from build123d import *

# Parameters (mm, degrees)
SKETCH_1_W                   = 160
SKETCH_1_H                   = 120
EXTRUDE_1_DEPTH              = 4
SKETCH_2_R                   = 4
SKETCH_2_R_2                 = 2.65
SKETCH_2_R_3                 = 6.75
CUT_EXTRUDE_1_DEPTH          = 24
CUT_EXTRUDE_2_DEPTH          = 54
SKETCH_5_R                   = 1.525
CUT_EXTRUDE_3_DEPTH          = 54
CUT_EXTRUDE_4_DEPTH          = 84
FILLET_1_R                   = 10
HOLE_WIZARD_M3_1_D           = 3.05
HOLE_WIZARD_M3_1_DEPTH       = 7.5
HOLE_WIZARD_M3_1_CSINK_D     = 6.6
HOLE_WIZARD_M3_1_CSINK_ANGLE = 90
HOLE_WIZARD_M3_1_TIP         = 0.916312444
FILLET_2_R                   = 2


with BuildPart() as part:
    # 草图1 → 凸台-拉伸1 (new body)
    with BuildSketch(Plane.XY):
        Rectangle(SKETCH_1_W, SKETCH_1_H)
    extrude(amount=EXTRUDE_1_DEPTH)

    # 草图2 → 切除-拉伸1 (cut)
    with BuildSketch(Plane(origin=(0, 0, 0), x_dir=(-1, 0, 0), z_dir=(0, 0, -1))):
        with Locations((-47.5, 38)):
            Circle(SKETCH_2_R)
        with Locations((-56.749921469, 44.53912734)):
            Circle(SKETCH_2_R_2)
        with Locations((-69.194904497, 52.913039057)):
            Circle(SKETCH_2_R_2)
        with Locations((-27.711627738, 25)):
            Circle(SKETCH_2_R_2)
        with Locations((-10, 25)):
            Circle(SKETCH_2_R_3)
    cut_extrude_1 = extrude(amount=-CUT_EXTRUDE_1_DEPTH, mode=Mode.SUBTRACT)

    # 镜向1: 切除-拉伸1 across plane
    add(cut_extrude_1.mirror(Plane(origin=(0, 0, 0), x_dir=(0, 0, 1), z_dir=(1, 0, 0))), mode=Mode.SUBTRACT)

    # 草图3 → 切除-拉伸2 (cut)
    with BuildSketch(Plane(origin=(0, 0, 0), x_dir=(-1, 0, 0), z_dir=(0, 0, -1))):
        Polygon((-61.851610318, 60), (-40.030198451, 45), (40.030198451, 45), (61.851610318, 60), align=None)
    extrude(amount=-CUT_EXTRUDE_2_DEPTH, mode=Mode.SUBTRACT)

    # 草图5 → 切除-拉伸3 (cut)
    with BuildSketch(Plane(origin=(0, 0, 0), x_dir=(-1, 0, 0), z_dir=(0, 0, -1))):
        with Locations((-20.859650045, 35.859650045)):
            Circle(SKETCH_5_R)
        with Locations((-20.859650045, -5.859650045)):
            Circle(SKETCH_5_R)
        with Locations((20.859650045, -5.859650045)):
            Circle(SKETCH_5_R)
        with Locations((20.859650045, 35.859650045)):
            Circle(SKETCH_5_R)
    extrude(amount=-CUT_EXTRUDE_3_DEPTH, mode=Mode.SUBTRACT)

    # 草图6 → 切除-拉伸4 (cut)
    with BuildSketch(Plane(origin=(0, 0, 0), x_dir=(-1, 0, 0), z_dir=(0, 0, -1))):
        with BuildLine():
            Line((-80, 50), (-28.863438287, -9.71643037))
            ThreePointArc((-28.863438287, -9.71643037), (0, -23), (28.863438287, -9.71643037))
            Line((28.863438287, -9.71643037), (80, 50))
            Line((80, 50), (80, -60))
            Line((80, -60), (-80, -60))
            Line((-80, -60), (-80, 50))
        make_face()
    extrude(amount=-CUT_EXTRUDE_4_DEPTH, mode=Mode.SUBTRACT)

    # 圆角1
    fillet_1_edges = [part.edges().sort_by_distance(p)[0] for p in [
        (-80, 60, 2),
        (80, 60, 2),
    ]]
    fillet(fillet_1_edges, radius=FILLET_1_R - 0.0001)  # a hair under: the kernel refuses the full size

    # M3 十字槽半沉头木螺钉的锥形沉头孔1
    with Locations(Plane.XY.offset(4)):
        with Locations((-20.859650045, 35.859650045), (20.859650045, 35.859650045), (20.859650045, -5.859650045), (-20.859650045, -5.859650045)):
            CounterSinkHole(HOLE_WIZARD_M3_1_D / 2, HOLE_WIZARD_M3_1_CSINK_D / 2, depth=HOLE_WIZARD_M3_1_DEPTH, counter_sink_angle=HOLE_WIZARD_M3_1_CSINK_ANGLE)
            with Locations((0, 0, -(HOLE_WIZARD_M3_1_DEPTH + HOLE_WIZARD_M3_1_TIP / 2))):  # 118° drill point
                Cone(0, HOLE_WIZARD_M3_1_D / 2, HOLE_WIZARD_M3_1_TIP, mode=Mode.SUBTRACT)

    # 圆角2
    fillet_2_edges = [part.edges().sort_by_distance(p)[0] for p in [
        (80, 50, 2),
        (-80, 50, 2),
        (61.851610318, 60, 2),
        (-61.851610318, 60, 2),
        (-40.030198451, 45, 2),
        (40.030198451, 45, 2),
    ]]
    fillet(fillet_2_edges, radius=FILLET_2_R)


solid = part.part
Part model, mm, in its own coordinate system. A direction names the side the tool comes from. Coordinates: 2 decimals unless noted, no trailing zeros. Order: outer loops, then holes, each group sorted by start corner. A loop starts at its lowest first (then second) coordinate and runs counter-clockwise, first axis right, second up. Notation, with made-up numbers: (56.5, -2.75) - (76.5, -2.75) arc R24 ccw to (76.5, 10.25) - close; hole circle Ø1 at (60, -2.75). An arc over 180 degrees is marked (long way). Use CSV: the item, a comma, the result in double quotes.
Item 1: Mould opens along X. For faces 1 (the face through (-1, 19, 4)), 2 (the face through (-76.829, 57.305, 2.028)), 3 (the face through (-50.795, 52.4, 1.972)) say: +X half, -X half, draft (parallel to the pull), parting line (faces both ways), or undercut.
Solved:
face 1,"draft"
face 2,"-X half"
face 3,"undercut"
Item 2: Saw through at C-C on x = 47.5. Give the cut face in (y, z).
Solved:
outline,"(12.05, 0) - (34, 0) - (34, 4) - (12.05, 4) - close; (42, 0) - (50.13, 0) - (50.13, 4) - (42, 4) - close"
Item 3: Drop a flat-ended pin along its axis: P1, Ø13, axis at x = 47.5, y = 38, coming from the -Z side. Give the stop position or say it passes through.
Solved:
P1,"stops at z = 0"
Item 4: Saw through at D-D on z = 1.45. Give the number of separate pieces and of enclosed holes in the cut face, and give its area (3 significant figures).
Solved:
separate pieces,"1"
enclosed holes,"14"
area,"6,510 mm²"
Item 5: Saw through at B-B on y = 25. Give the cut face in (x, z), and give its area (3 significant figures).
Solved:
outline,"(-58.59, 0) - (-30.36, 0) - (-30.36, 4) - (-58.59, 4) - close; (-25.06, 0) - (-16.75, 0) - (-16.75, 4) - (-25.06, 4) - close; (-3.25, 0) - (3.25, 0) - (3.25, 4) - (-3.25, 4) - close; (16.75, 0) - (25.06, 0) - (25.06, 4) - (16.75, 4) - close; (30.36, 0) - (58.59, 0) - (58.59, 4) - (30.36, 4) - close"
area,"318 mm²"
Item 6: Probe probe 1 along X at (y, z) = (26, 2.05); probe 2 along Y at (x, z) = (-20, 0.45); probe 3 along X at (y, z) = (20.5, 0.65). List the from-to ranges inside material, lowest first.
Solved:
probe 1,"x = -59.45 to -30.17, -25.26 to -16.68, -3.32 to 3.32, 16.68 to 25.26, 30.17 to 59.45"
probe 2,"y = -17.31 to -7.12, -4.6 to 34.6, 37.12 to 45"
probe 3,"x = -54.74 to -15.03, -4.97 to 4.97, 15.03 to 54.74"
Item 7: Saw through at A-A on x = 10. Give the cut face in (y, z), and give its area (3 significant figures).
Solved:
outline,"(-21.66, 0) - (18.25, 0) - (18.25, 4) - (-21.66, 4) - close; (31.75, 0) - (45, 0) - (45, 4) - (31.75, 4) - close"
area,"213 mm²"
Item 8: 3-axis set-ups, long thin cutter, end or side, ignore diameter. For faces 4 (the face through (-3.562, 27.028, 1.972)), 5 (the face through (51.086, 52.6, 1.972)): which of +Z, -Z, +X, -X, +Y, -Y reach the whole face in a straight line?
Solved:
face 4,"+Z, -Z"
face 5,"+Z, -Z, +Y"
